CAD build for the part. Positions are in the model's coordinates, mm. A direction names the side the tool comes from. Give positions to 0.01 mm unless a question says otherwise; leave off trailing zeros. Write each loop counter-clockwise with the first axis right and the second up, starting at its lowest first coordinate (ties: lowest second). Pieces come first, ordered by that corner, then holes. Notation, with made-up numbers: (-31, 86) - (23, 86) arc R14 ccw to (23, 97) - close; hole circle Ø9 at (40.25, -32). An arc over 180 degrees is marked (long way). Write item = value, one per line. Start each with the question number.
```python
from build123d import *

# Parameters (mm, degrees)
SKETCH_1_R      = 4
SKETCH_1_R_2    = 11.5
SKETCH_1_R_3    = 1.5
EXTRUDE_1_DEPTH = 5


with BuildPart() as part:
    # 草图1 → 凸台-拉伸1 (new body)
    with BuildSketch(Plane(origin=(0, 0, 0), x_dir=(0, 0, -1), z_dir=(1, 0, 0))):
        with BuildLine():
            Line((-69.746431282, -6.912239682), (-69.746431282, -3.912239682))
            ThreePointArc((-69.746431282, -3.912239682), (-69.160644844, -2.49802612), (-67.746431282, -1.912239682))
            Line((-67.746431282, -1.912239682), (78.253568718, -1.912239682))
            ThreePointArc((78.253568718, -1.912239682), (79.667782281, -2.49802612), (80.253568718, -3.912239682))
            Line((80.253568718, -3.912239682), (80.253568718, -6.912239682))
            ThreePointArc((80.253568718, -6.912239682), (81.718034813, -10.447773588), (85.253568718, -11.912239682))
            Line((85.253568718, -11.912239682), (125.253568718, -11.912239682))
            ThreePointArc((125.253568718, -11.912239682), (128.789102624, -10.447773588), (130.253568718, -6.912239682))
            Line((130.253568718, -6.912239682), (130.253568718, 25.387760318))
            Line((130.253568718, 25.387760318), (125.253568718, 25.387760318))
            Line((125.253568718, 25.387760318), (125.253568718, 45.387760318))
            Line((125.253568718, 45.387760318), (130.253568718, 45.387760318))
            Line((130.253568718, 45.387760318), (130.253568718, 65.387760318))
            Line((130.253568718, 65.387760318), (125.253568718, 65.387760318))
            Line((125.253568718, 65.387760318), (125.253568718, 85.387760318))
            Line((125.253568718, 85.387760318), (130.253568718, 85.387760318))
            Line((130.253568718, 85.387760318), (130.253568718, 105.387760318))
            Line((130.253568718, 105.387760318), (120.253568718, 105.387760318))
            ThreePointArc((120.253568718, 105.387760318), (118.132248375, 104.509080662), (117.253568718, 102.387760318))
            Line((117.253568718, 102.387760318), (117.253568718, 93.387760318))
            ThreePointArc((117.253568718, 93.387760318), (116.374889062, 91.266439974), (114.253568718, 90.387760318))
            Line((114.253568718, 90.387760318), (105.253568718, 90.387760318))
            ThreePointArc((105.253568718, 90.387760318), (103.132248375, 91.266439974), (102.253568718, 93.387760318))
            Line((102.253568718, 93.387760318), (102.253568718, 102.387760318))
            ThreePointArc((102.253568718, 102.387760318), (101.374889062, 104.509080662), (99.253568718, 105.387760318))
            Line((99.253568718, 105.387760318), (-88.746431282, 105.387760318))
            ThreePointArc((-88.746431282, 105.387760318), (-90.867751625, 104.509080662), (-91.746431282, 102.387760318))
            Line((-91.746431282, 102.387760318), (-91.746431282, 93.387760318))
            ThreePointArc((-91.746431282, 93.387760318), (-92.625110938, 91.266439974), (-94.746431282, 90.387760318))
            Line((-94.746431282, 90.387760318), (-103.746431282, 90.387760318))
            ThreePointArc((-103.746431282, 90.387760318), (-105.867751625, 91.266439974), (-106.746431282, 93.387760318))
            Line((-106.746431282, 93.387760318), (-106.746431282, 102.387760318))
            ThreePointArc((-106.746431282, 102.387760318), (-107.625110938, 104.509080662), (-109.746431282, 105.387760318))
            Line((-109.746431282, 105.387760318), (-119.746431282, 105.387760318))
            Line((-119.746431282, 105.387760318), (-119.746431282, 85.387760318))
            Line((-119.746431282, 85.387760318), (-114.746431282, 85.387760318))
            Line((-114.746431282, 85.387760318), (-114.746431282, 65.387760318))
            Line((-114.746431282, 65.387760318), (-119.746431282, 65.387760318))
            Line((-119.746431282, 65.387760318), (-119.746431282, 45.387760318))
            Line((-119.746431282, 45.387760318), (-114.746431282, 45.387760318))
            Line((-114.746431282, 45.387760318), (-114.746431282, 25.387760318))
            Line((-114.746431282, 25.387760318), (-119.746431282, 25.387760318))
            Line((-119.746431282, 25.387760318), (-119.746431282, -6.912239682))
            ThreePointArc((-119.746431282, -6.912239682), (-118.281965187, -10.447773588), (-114.746431282, -11.912239682))
            Line((-114.746431282, -11.912239682), (-74.746431282, -11.912239682))
            ThreePointArc((-74.746431282, -11.912239682), (-71.210897376, -10.447773588), (-69.746431282, -6.912239682))
        make_face()
        with Locations((48.253568718, 96.387760318)):
            Circle(SKETCH_1_R, mode=Mode.SUBTRACT)
        with Locations((-37.746431282, 96.387760318)):
            Circle(SKETCH_1_R, mode=Mode.SUBTRACT)
        with Locations((5.253568718, 83.387760318)):
            Circle(SKETCH_1_R_2, mode=Mode.SUBTRACT)
        with Locations((-10.246431282, 98.887760318)):
            Circle(SKETCH_1_R_3, mode=Mode.SUBTRACT)
        with Locations((20.753568718, 98.887760318)):
            Circle(SKETCH_1_R_3, mode=Mode.SUBTRACT)
        with Locations((20.753568718, 67.887760318)):
            Circle(SKETCH_1_R_3, mode=Mode.SUBTRACT)
        with Locations((-10.246431282, 68.825049391)):
            Circle(SKETCH_1_R_3, mode=Mode.SUBTRACT)
        with Locations((127.753568718, 95.387760318)):
            Circle(SKETCH_1_R_3, mode=Mode.SUBTRACT)
        with Locations((127.753568718, 55.387760318)):
            Circle(SKETCH_1_R_3, mode=Mode.SUBTRACT)
        with Locations((-117.246431282, 95.387760318)):
            Circle(SKETCH_1_R_3, mode=Mode.SUBTRACT)
        with Locations((-117.246431282, 55.387760318)):
            Circle(SKETCH_1_R_3, mode=Mode.SUBTRACT)
    extrude(amount=EXTRUDE_1_DEPTH)


solid = part.part
```
1. Cut at B-B (x = 2.85). Count the separate pieces of the cut face and the enclosed holes in it, then the cut area to 3 significant figures.
2. Tool access for faces 4 (the flat face through (2, 25.388, 117)), 5 (the flat face through (2, 85.388, -128)), 6 (the cylindrical face through (2.465, -10.486, 71.25)), 7 (the flat face through (2, 98, 91.746)): list every direction of +Z, -Z, +X, -X, +Y, -Y with a clear straight run to the whole face (end or side of a thin tool).
3. Cut at C-C (z = -48.5). Give the cut face in (x, y), then the cut area to 3 significant figures.
4. Mould opens along Y. For faces 1 (the flat face through (2, 65.388, -128)), 2 (the flat face through (2, 105.388, -7)), 3 (the cylindrical face through (2.46, -10.41, 118.32)) say: +Y half, -Y half, draft (parallel to the pull), parting line (faces both ways), or undercut.
5. Cut at A-A (z = 38.5). Give the cut face in (x, y), then the cut area to 3 significant figures.
6. Wall check: line 1 along Z through (x, y) = (1.8, -6); line 2 along Y through (x, z) = (2.4, -70.5); line 3 along Z through (x, y) = (2.4, 33). Give the ranges that are in metal, low to high.
7. Pin check, flat tips, straight feed: pin 1 Ø10.5 at (y, z) = (96.39, -48.25) entering from -X; pin 2 Ø1.5 at (x, z) = (3.5, -127) entering from -Y; pin 3 Ø1.5 at (x, z) = (1.5, -112) entering from +Y; pin 4 Ø1.5 at (x, y) = (1.5, 40.5) entering from +Z. Stop position of each tip, or through.
Output:
q1.separate_pieces = 1
q1.enclosed_holes = 11
q1.area = 26,400 mm2
q2.face_4 = +Z, +X, -X
q2.face_5 = -Z, +X, -X
q2.face_6 = +X, -X, -Y
q2.face_7 = +X, -X, +Y
q3.outline = (0, -1.91) - (5, -1.91) - (5, 92.4) - (0, 92.4) - close; (0, 100.38) - (5, 100.38) - (5, 105.39) - (0, 105.39) - close
q3.area = 497 mm2
q4.face_1 = undercut
q4.face_2 = +Y half
q4.face_3 = -Y half
q5.outline = (0, -1.91) - (5, -1.91) - (5, 92.46) - (0, 92.46) - close; (0, 100.32) - (5, 100.32) - (5, 105.39) - (0, 105.39) - close
q5.area = 497 mm2
q6.line_1 = -130.25 to -80.25, 69.75 to 119.75
q6.line_2 = -1.91 to 105.39
q6.line_3 = -125.25 to 114.75
q7.pin_1 = 0
q7.pin_2 = -11.81
q7.pin_3 = 90.39
q7.pin_4 = 114.75
